Design review of the part built by this model. Coordinates are the model's own, in mm. A direction names the side the tool comes from. Coordinates: 2 decimals unless noted, no trailing zeros. Write each loop counter-clockwise with the first axis right and the second up, starting at its lowest first coordinate (ties: lowest second). Pieces come first, ordered by that corner, then holes.
Q1. For faces 4 (the flat face through (-12, 0, -2)), 5 (the flat face through (-2, 10, -9)), 6 (the flat face through (-2, -14, -13)), 7 (the flat face through (-2, 17, -20)), list the 3-axis set-ups (+Z, -Z, +X, -X, +Y, -Y) from which the entire face can be reached by the end or side of a thin tool; tool diameter is ignored.
Q2. The part is to be moulded in two halves that separate along Z. For faces 1 (the cylindrical face through (-15.7, 18.48, -21.81)), 2 (the flat face through (-2, -17, -20)), 3 (the flat face through (-2, 0, -16)), say which applies: released by +Z, released by -Z, zero draft, split by the parting line, or undercut.
Q3. Take a section at B-B, the plane x = 0. Write out the cut boundary in (y, z), plus the area to 3 significant figures.
Q4. Take a section at A-A, the plane z = -18. Write out the cut boundary in (x, y), plus the area to 3 significant figures.
Q5. For pin 1 Ø1.5 at (x, y) = (-6.5, 1) entering from -Z; pin 2 Ø20 at (x, z) = (4.5, 0.5) entering from -Y; pin 3 Ø10 at (x, z) = (0.5, 3) entering from +Y, all flat-tipped, find the tip position at first contact; note any pin that passes through.
Q6. Take a section at C-C, the plane y = -1. Write out the cut boundary in (x, z), plus the area to 3 significant figures.
Q7. For L1, parallel to Y at x = -6.5, z = -18.5; L2, parallel to X at y = -19, z = -20; L3, parallel to Z at x = 12, y = 16, list the stretches that pass through material, from the lowest coordinate up.
Q8. Take a section at D-D, the plane z = -7. Write out the cut boundary in (x, y), plus the area to 3 significant figures.
from build123d import *

# Parameters (mm, degrees)
F1_DEPTH = 10
F0_W     = 36
F0_H     = 10.5
F2_DEPTH = 20
F3_W     = 34
F3_H     = 7.5
F4_DEPTH = 36.001
F5_R     = 1.25
F6_DEPTH = 43.8
F7_SIZE  = 3
F8_SIZE  = 2


with BuildPart() as f1:
    # F0 (on Front) → F1 (new body, symmetric)
    with BuildSketch(Plane.XZ):
        with BuildLine():
            ThreePointArc((-8, 0), (0, 8), (8, 0))
            Line((8, 0), (12, 0))
            ThreePointArc((12, 0), (0, 12), (-12, 0))
            Line((-12, 0), (-8, 0))
        make_face()
        with BuildLine():
            Line((12, 0), (8, 0))
            ThreePointArc((8, 0), (0, -8), (-8, 0))
            Line((-8, 0), (-12, 0))
            Line((-12, 0), (-12, -3.318))
            ThreePointArc((-12, -3.318), (-14.1841212285, -9.5264890007), (-19.774330755, -13))
            Line((-19.774330755, -13), (16.225669245, -13))
            ThreePointArc((16.225669245, -13), (13.1191975203, -9.4390615485), (12, -4.848))
            Line((12, -4.848), (12, 0))
        make_face()
    extrude(amount=F1_DEPTH, both=True)

    # F0 (on Front) → F2 (join, symmetric)
    with BuildSketch(Plane.XZ):
        with Locations((-1.774330755, -18.25)):
            Rectangle(F0_W, F0_H)
    extrude(amount=F2_DEPTH, both=True)

    # F3 (on face) → F4 (cut, through all)
    with BuildSketch(Plane(origin=(-19.774330755, 0, 0), x_dir=(0, -1, 0), z_dir=(-1, 0, 0))):
        with Locations((0, -19.75)):
            Rectangle(F3_W, F3_H)
    extrude(amount=-F4_DEPTH, mode=Mode.SUBTRACT)

    # F5 (on face) → F6 (cut)
    with BuildSketch(Plane.XZ.offset(20)):
        with Locations((-16.274330755, -20.7)):
            Circle(F5_R)
        with Locations((5.725669245, -20.7)):
            Circle(F5_R)
    extrude(amount=-F6_DEPTH, mode=Mode.SUBTRACT)

    # F7
    f7_edges = [f1.edges().sort_by_distance(p)[0] for p in [
        (-19.774331, -18.5, -23.5),
        (-19.774331, 18.5, -23.5),
        (16.225669, 18.5, -23.5),
        (16.225669, -18.5, -23.5),
    ]]
    chamfer(f7_edges, length=F7_SIZE)

    # F8
    f8_edges = [f1.edges().sort_by_distance(p)[0] for p in [
        (-1.774331, -20, -13),
        (-1.774331, 20, -13),
    ]]
    chamfer(f8_edges, length=F8_SIZE)


solid = f1.part
Responses:
1. face 4: +Z, -X, +Y, -Y
1. face 5: +Z, +X, -X, +Y
1. face 6: +Z, +X, -X, -Y
1. face 7: -Z, +X, -X
2. face 1: undercut
2. face 2: zero draft
2. face 3: released by -Z
3. outline: (-20, -23.5) - (-17, -23.5) - (-17, -16) - (17, -16) - (17, -23.5) - (20, -23.5) - (20, -15) - (18, -13) - (10, -13) - (10, -8) - (-10, -8) - (-10, -13) - (-18, -13) - (-20, -15) - close; (-10, 8) - (10, 8) - (10, 12) - (-10, 12) - close
3. area: 341 mm2
4. outline: (-19.77, -20) - (16.23, -20) - (16.23, -17) - (-19.77, -17) - close; (-19.77, 17) - (16.23, 17) - (16.23, 20) - (-19.77, 20) - close
4. area: 216 mm2
5. pin 1: stops at z = -16
5. pin 2: stops at y = -10
5. pin 3: stops at y = 10
6. outline: (-19.77, -16) - (16.23, -16) - (16.23, -13) arc R9.98 cw to (12, -4.85) - (12, 0) arc R12 ccw to (-12, 0) - (-12, -3.32) arc R9.92 cw to (-19.77, -13) - close; hole circle Ø16 at (0, 0)
6. area: 475 mm2
7. L1: y = -20 to -17, 17 to 20
7. L2: x = -19.77 to -17.31, -15.24 to 4.69, 6.76 to 16.23
7. L3: z = -16 to -13
8. outline: (-12.71, -10) - (-3.87, -10) - (-3.87, 10) - (-12.71, 10) - close; (3.87, -10) - (12.23, -10) - (12.23, 10) - (3.87, 10) - close
8. area: 344 mm2
